For this review, take the finished solid that the model builds, in its own axes (mm). Face numbers are marked on the shaded views. A direction names the side the tool comes from. Round coordinates to 2 decimals unless told otherwise and drop trailing zeros. Loops run counter-clockwise (first coordinate to the right, second up) from the corner with the lowest first, then second, coordinate; pieces in that order, holes last. Notation, with made-up numbers: (-32, 60.25) -> (-19, 60.25) arc R9 ccw to (-19, 68.25) -> close; hole circle Ø6 at (69.5, -23). An arc over 180 degrees is marked (long way). Write each question's results on one line, items separated by ' | '.
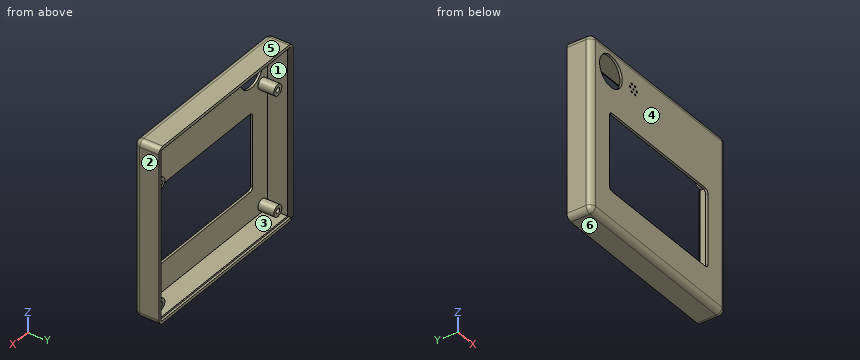
```python
from build123d import *

# Parameters (mm, degrees)
SKETCH3_W           = 101
SKETCH3_H           = 95
BOSS_EXTRUDE2_DEPTH = 1.2
SKETCH5_W           = 101
SKETCH5_H           = 95
SKETCH5_W_2         = 96
SKETCH5_H_2         = 90
BOSS_EXTRUDE3_DEPTH = 11
SKETCH6_W           = 101
SKETCH6_H           = 95
SKETCH6_W_2         = 97.8
SKETCH6_H_2         = 91.8
BOSS_EXTRUDE4_DEPTH = 1.2
FILLET1_R           = 3
SKETCH7_R           = 3
BOSS_EXTRUDE5_DEPTH = 8.6
SKETCH8_R           = 1.4
CUT_EXTRUDE1_DEPTH  = 7
CUT_EXTRUDE2_REACH  = 3.2
SKETCH9_R           = 8.5
SKETCH9_R_2         = 0.5


with BuildPart() as part:
    # Sketch3 → Boss-Extrude2 (new body)
    with BuildSketch(Plane(origin=(0, 0, 0), x_dir=(1, 0, 0), z_dir=(0, 1, 0))):
        with Locations((46.5, 43.5)):
            Rectangle(SKETCH3_W, SKETCH3_H)
    extrude(amount=BOSS_EXTRUDE2_DEPTH)

    # Sketch5 → Boss-Extrude3 (add)
    with BuildSketch(Plane(origin=(0, 1.2, 0), x_dir=(1, 0, 0), z_dir=(0, 1, 0))):
        with Locations((46.5, 43.5)):
            Rectangle(SKETCH5_W, SKETCH5_H)
        with Locations((46.5, 43.5)):
            Rectangle(SKETCH5_W_2, SKETCH5_H_2, mode=Mode.SUBTRACT)
    extrude(amount=BOSS_EXTRUDE3_DEPTH)

    # Sketch6 → Boss-Extrude4 (add)
    with BuildSketch(Plane(origin=(0, 12.2, 0), x_dir=(1, 0, 0), z_dir=(0, 1, 0))):
        with Locations((46.5, 43.5)):
            Rectangle(SKETCH6_W, SKETCH6_H)
        with Locations((46.5, 43.5)):
            Rectangle(SKETCH6_W_2, SKETCH6_H_2, mode=Mode.SUBTRACT)
    extrude(amount=BOSS_EXTRUDE4_DEPTH)

    # Fillet1
    fillet1_edges = [part.edges().sort_by_distance(p)[0] for p in [
        (46.5, 0, -91),
        (97, 0, -43.5),
        (46.5, 0, 4),
        (-4, 0, -43.5),
        (-4, 6.7, -91),
        (97, 6.7, -91),
        (97, 6.7, 4),
        (-4, 6.7, 4),
    ]]
    fillet(fillet1_edges, radius=FILLET1_R)

    # Sketch7 → Boss-Extrude5 (add)
    with BuildSketch(Plane(origin=(0, 1.2, 0), x_dir=(1, 0, 0), z_dir=(0, 1, 0))):
        with Locations((2.5, 84.5)):
            Circle(SKETCH7_R)
        with Locations((90.5, 84.5)):
            Circle(SKETCH7_R)
        with Locations((90.5, 19.5)):
            Circle(SKETCH7_R)
        with Locations((2.5, 19.5)):
            Circle(SKETCH7_R)
    extrude(amount=BOSS_EXTRUDE5_DEPTH)

    # Sketch8 → Cut-Extrude1 (cut)
    with BuildSketch(Plane(origin=(0, 9.8, 0), x_dir=(1, 0, 0), z_dir=(0, 1, 0))):
        with Locations((2.5, 84.5)):
            Circle(SKETCH8_R)
        with Locations((90.5, 84.5)):
            Circle(SKETCH8_R)
        with Locations((90.5, 19.5)):
            Circle(SKETCH8_R)
        with Locations((2.5, 19.5)):
            Circle(SKETCH8_R)
    extrude(amount=-CUT_EXTRUDE1_DEPTH, mode=Mode.SUBTRACT)

    # Sketch9 → Cut-Extrude2 (cut, up to next)
    with BuildSketch(Plane(origin=(0, 1.2, 0), x_dir=(1, 0, 0), z_dir=(0, 1, 0)), mode=Mode.PRIVATE) as cut_extrude2_sk1:
        with Locations((10.5, 9)):
            Circle(SKETCH9_R)
    cut_extrude2_tool1 = extrude(cut_extrude2_sk1.sketch, amount=-CUT_EXTRUDE2_REACH, mode=Mode.PRIVATE) & part.part
    add(cut_extrude2_tool1.solids().sort_by_distance((10.5, 1.2, -9))[0], mode=Mode.SUBTRACT)
    # Sketch9 → Cut-Extrude2 (cut, up to next)
    with BuildSketch(Plane(origin=(0, 1.2, 0), x_dir=(1, 0, 0), z_dir=(0, 1, 0)), mode=Mode.PRIVATE) as cut_extrude2_sk2:
        with Locations((27.5, 9)):
            Circle(SKETCH9_R_2)
    cut_extrude2_tool2 = extrude(cut_extrude2_sk2.sketch, amount=-CUT_EXTRUDE2_REACH, mode=Mode.PRIVATE) & part.part
    add(cut_extrude2_tool2.solids().sort_by_distance((27.5, 1.2, -9))[0], mode=Mode.SUBTRACT)
    # Sketch9 → Cut-Extrude2 (cut, up to next)
    with BuildSketch(Plane(origin=(0, 1.2, 0), x_dir=(1, 0, 0), z_dir=(0, 1, 0)), mode=Mode.PRIVATE) as cut_extrude2_sk3:
        with Locations((28.75, 11.165063509)):
            Circle(SKETCH9_R_2)
    cut_extrude2_tool3 = extrude(cut_extrude2_sk3.sketch, amount=-CUT_EXTRUDE2_REACH, mode=Mode.PRIVATE) & part.part
    add(cut_extrude2_tool3.solids().sort_by_distance((28.75, 1.2, -11.165064))[0], mode=Mode.SUBTRACT)
    # Sketch9 → Cut-Extrude2 (cut, up to next)
    with BuildSketch(Plane(origin=(0, 1.2, 0), x_dir=(1, 0, 0), z_dir=(0, 1, 0)), mode=Mode.PRIVATE) as cut_extrude2_sk4:
        with Locations((26.25, 11.165063509)):
            Circle(SKETCH9_R_2)
    cut_extrude2_tool4 = extrude(cut_extrude2_sk4.sketch, amount=-CUT_EXTRUDE2_REACH, mode=Mode.PRIVATE) & part.part
    add(cut_extrude2_tool4.solids().sort_by_distance((26.25, 1.2, -11.165064))[0], mode=Mode.SUBTRACT)
    # Sketch9 → Cut-Extrude2 (cut, up to next)
    with BuildSketch(Plane(origin=(0, 1.2, 0), x_dir=(1, 0, 0), z_dir=(0, 1, 0)), mode=Mode.PRIVATE) as cut_extrude2_sk5:
        with Locations((25, 9)):
            Circle(SKETCH9_R_2)
    cut_extrude2_tool5 = extrude(cut_extrude2_sk5.sketch, amount=-CUT_EXTRUDE2_REACH, mode=Mode.PRIVATE) & part.part
    add(cut_extrude2_tool5.solids().sort_by_distance((25, 1.2, -9))[0], mode=Mode.SUBTRACT)
    # Sketch9 → Cut-Extrude2 (cut, up to next)
    with BuildSketch(Plane(origin=(0, 1.2, 0), x_dir=(1, 0, 0), z_dir=(0, 1, 0)), mode=Mode.PRIVATE) as cut_extrude2_sk6:
        with Locations((26.25, 6.834936491)):
            Circle(SKETCH9_R_2)
    cut_extrude2_tool6 = extrude(cut_extrude2_sk6.sketch, amount=-CUT_EXTRUDE2_REACH, mode=Mode.PRIVATE) & part.part
    add(cut_extrude2_tool6.solids().sort_by_distance((26.25, 1.2, -6.834936))[0], mode=Mode.SUBTRACT)
    # Sketch9 → Cut-Extrude2 (cut, up to next)
    with BuildSketch(Plane(origin=(0, 1.2, 0), x_dir=(1, 0, 0), z_dir=(0, 1, 0)), mode=Mode.PRIVATE) as cut_extrude2_sk7:
        with Locations((28.75, 6.834936491)):
            Circle(SKETCH9_R_2)
    cut_extrude2_tool7 = extrude(cut_extrude2_sk7.sketch, amount=-CUT_EXTRUDE2_REACH, mode=Mode.PRIVATE) & part.part
    add(cut_extrude2_tool7.solids().sort_by_distance((28.75, 1.2, -6.834936))[0], mode=Mode.SUBTRACT)
    # Sketch9 → Cut-Extrude2 (cut, up to next)
    with BuildSketch(Plane(origin=(0, 1.2, 0), x_dir=(1, 0, 0), z_dir=(0, 1, 0)), mode=Mode.PRIVATE) as cut_extrude2_sk8:
        with Locations((30, 9)):
            Circle(SKETCH9_R_2)
    cut_extrude2_tool8 = extrude(cut_extrude2_sk8.sketch, amount=-CUT_EXTRUDE2_REACH, mode=Mode.PRIVATE) & part.part
    add(cut_extrude2_tool8.solids().sort_by_distance((30, 1.2, -9))[0], mode=Mode.SUBTRACT)
    # Sketch9 → Cut-Extrude2 (cut, up to next)
    with BuildSketch(Plane(origin=(0, 1.2, 0), x_dir=(1, 0, 0), z_dir=(0, 1, 0)), mode=Mode.PRIVATE) as cut_extrude2_sk9:
        with BuildLine():
            Line((11.5, 31), (81.5, 31))
            ThreePointArc((81.5, 31), (82.914213562, 31.585786438), (83.5, 33))
            Line((83.5, 33), (83.5, 71))
            ThreePointArc((83.5, 71), (82.914213562, 72.414213562), (81.5, 73))
            Line((81.5, 73), (11.5, 73))
            ThreePointArc((11.5, 73), (10.085786438, 72.414213562), (9.5, 71))
            Line((9.5, 71), (9.5, 33))
            ThreePointArc((9.5, 33), (10.085786438, 31.585786438), (11.5, 31))
        make_face()
    cut_extrude2_tool9 = extrude(cut_extrude2_sk9.sketch, amount=-CUT_EXTRUDE2_REACH, mode=Mode.PRIVATE) & part.part
    add(cut_extrude2_tool9.solids().sort_by_distance((46.5, 1.2, -52))[0], mode=Mode.SUBTRACT)


solid = part.part
```
1. Consider section C-C (z = -27). State the section outline as (x, y) points, plus the area to 3 significant figures.
Values found:
outline: (-4, 3) arc R3 ccw to (-1, 0) -> (94, 0) arc R3 ccw to (97, 3) -> (97, 13.4) -> (95.4, 13.4) -> (95.4, 12.2) -> (94.5, 12.2) -> (94.5, 1.2) -> (-1.5, 1.2) -> (-1.5, 12.2) -> (-2.4, 12.2) -> (-2.4, 13.4) -> (-4, 13.4) -> close | area: 176 mm2
2. For pin 1 (0.8 mm diameter, centred on x = 90.5, z = -20, fed in from +Y); pin 2 (3 mm diameter, centred on x = 3, z = -85, fed in from +Y); pin 3 (6.5 mm diameter, centred on x = 91.5, z = -20.5, fed in from +Y); pin 4 (12 mm diameter, centred on x = 76, z = -52.5, fed in from +Y), all flat-tipped, find the tip position at first contact; note any pin that passes through.
Values found:
pin 1: stops at y = 2.8 | pin 2: stops at y = 9.8 | pin 3: stops at y = 12.2 | pin 4: passes through
3. Consider section B-B (x = 52). State the section outline as (y, z) points.
Values found:
outline: (0, -88) arc R3 ccw to (3, -91) -> (13.4, -91) -> (13.4, -89.4) -> (12.2, -89.4) -> (12.2, -88.5) -> (1.2, -88.5) -> (1.2, -73) -> (0, -73) -> close; (0, -31) -> (1.2, -31) -> (1.2, 1.5) -> (12.2, 1.5) -> (12.2, 2.4) -> (13.4, 2.4) -> (13.4, 4) -> (3, 4) arc R3 ccw to (0, 1) -> close
4. Consider section A-A (z = -69.5). State the section outline as (x, y) points.
Values found:
outline: (-4, 3) arc R3 ccw to (-1, 0) -> (9.5, 0) -> (9.5, 1.2) -> (-1.5, 1.2) -> (-1.5, 12.2) -> (-2.4, 12.2) -> (-2.4, 13.4) -> (-4, 13.4) -> close; (83.5, 0) -> (94, 0) arc R3 ccw to (97, 3) -> (97, 13.4) -> (95.4, 13.4) -> (95.4, 12.2) -> (94.5, 12.2) -> (94.5, 1.2) -> (83.5, 1.2) -> close
5. To check wall thickness, follow probe 1 along Z at (x, y) = (90.5, 7.5); probe 2 along X at (y, z) = (12.75, 0); probe 3 along X at (y, z) = (10.5, -20.5). State the ranges of each line that lie inside material, in increasing order.
Values found:
probe 1: z = -91 to -88.5, -87.5 to -85.9, -83.1 to -81.5, -22.5 to -20.9, -18.1 to -16.5, 1.5 to 4 | probe 2: x = -4 to -2.4, 95.4 to 97 | probe 3: x = -4 to -1.5, 94.5 to 97
6. Draft analysis for pull direction Z (two halves, no side actions). For the marked faces 3, 4, 5 and 6, state which applies: released by +Z, released by -Z, zero draft, split by the parting line, or undercut.
Values found:
face 3: undercut | face 4: zero draft | face 5: released by +Z | face 6: released by -Z
7. Tool access review of the marked faces 1 and 2: name each direction out of +Z, -Z, +X, -X, +Y, -Y from which nothing blocks a thin tool from reaching the whole face with its end or side.
Values found:
face 1: +Y | face 2: +Z, -Z, +X, +Y, -Y
